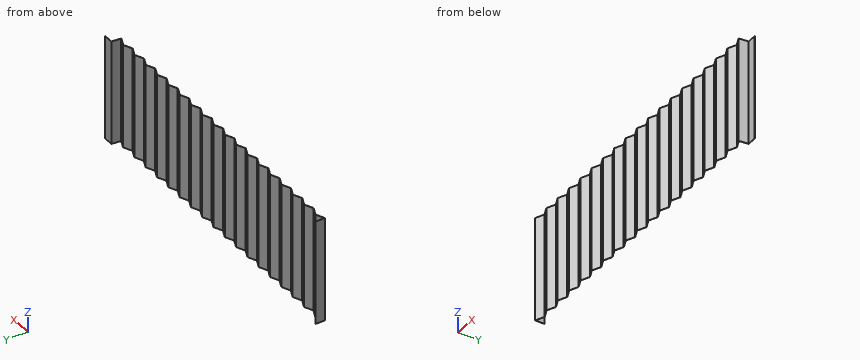
from build123d import *

# Parameters (mm, degrees)
EXTRUDE_THIN1_DEPTH = 85


with BuildPart() as part:
    # Sketch1 → Extrude-Thin1 (new, symmetric)
    with BuildSketch(Plane.XY):
        Polygon((0, 15.1), (0, 0), (13.79208513, 6.147226022), (27.58417026, 0), (41.37625539, 6.147226022), (55.16834052, 0), (68.960425651, 6.147226022), (82.752510781, 0), (96.544595911, 6.147226022), (110.336681041, 0), (124.128766171, 6.147226022), (137.920851301, 0), (151.712936431, 6.147226022), (165.505021561, 0), (179.297106692, 6.147226022), (193.089191822, 0), (206.881276952, 6.147226022), (220.673362082, 0), (234.465447212, 6.147226022), (248.257532342, 0), (262.049617472, 6.147226022), (275.841702602, 0), (289.633787732, 6.147226022), (303.425872863, 0), (317.217957993, 6.147226022), (331.010043123, 0), (344.802128253, 6.147226022), (358.594213383, 0), (372.386298513, 6.147226022), (386.178383643, 0), (399.970468773, 6.147226022), (413.762553904, 0), (427.554639034, 6.147226022), (441.346724164, 0), (455.138809294, 6.147226022), (468.930894424, 0), (482.722979554, 6.147226022), (496.515064684, 0), (498.249999842, 15), (513.249999842, 15), (513.249999842, 15.3), (497.982698545, 15.3), (496.263996817, 0.440351902), (482.722979554, 6.475675271), (468.930894424, 0.328449249), (455.138809294, 6.475675271), (441.346724164, 0.328449249), (427.554639034, 6.475675271), (413.762553904, 0.328449249), (399.970468773, 6.475675271), (386.178383643, 0.328449249), (372.386298513, 6.475675271), (358.594213383, 0.328449249), (344.802128253, 6.475675271), (331.010043123, 0.328449249), (317.217957993, 6.475675271), (303.425872863, 0.328449249), (289.633787732, 6.475675271), (275.841702602, 0.328449249), (262.049617472, 6.475675271), (248.257532342, 0.328449249), (234.465447212, 6.475675271), (220.673362082, 0.328449249), (206.881276952, 6.475675271), (193.089191822, 0.328449249), (179.297106692, 6.475675271), (165.505021561, 0.328449249), (151.712936431, 6.475675271), (137.920851301, 0.328449249), (124.128766171, 6.475675271), (110.336681041, 0.328449249), (96.544595911, 6.475675271), (82.752510781, 0.328449249), (68.960425651, 6.475675271), (55.16834052, 0.328449249), (41.37625539, 6.475675271), (27.58417026, 0.328449249), (13.79208513, 6.475675271), (0.3, 0.462161286), (0.3, 15.1), align=None)
    extrude(amount=EXTRUDE_THIN1_DEPTH, both=True)


solid = part.part
Geometry check sheet. Reference: the model listing, model coordinates, mm. Give positions to 0.01 mm unless a question says otherwise; leave off trailing zeros. Order: outer loops, then holes, each group sorted by start corner. A loop starts at its lowest first (then second) coordinate and runs counter-clockwise, first axis right, second up.
1) Gauge pin test, flat ends, axial feed: pin 1 (12 mm diameter, centred on x = 270.5, z = 62, fed in from -Y); pin 2 (7.5 mm diameter, centred on y = 9.5, z = -22.5, fed in from +X); pin 3 (2 mm diameter, centred on x = 196, z = 46.5, fed in from +Y); pin 4 (5 mm diameter, centred on x = 456.5, z = 10.5, fed in from +Y). Record the tip position at first contact, or that the pin passes through.
Results are:
pin 1: stops at y = 0
pin 2: stops at x = 498.05
pin 3: stops at y = 2.07
pin 4: stops at y = 6.48
2) Cross-section at A-A (y = 11). Record the boundary of the cut face in (x, z), then the cut area to 3 significant figures.
Results are:
outline: (0, -85) - (0.3, -85) - (0.3, 85) - (0, 85) - close; (497.49, -85) - (497.79, -85) - (497.79, 85) - (497.49, 85) - close
area: 102 mm2
3) Cross-section at B-B (x = 143.5). Record the boundary of the cut face in (y, z), then the cut area to 3 significant figures.
Results are:
outline: (2.49, -85) - (2.82, -85) - (2.82, 85) - (2.49, 85) - close
area: 55.8 mm2
4) Material ranges on probe 1 along X at (y, z) = (6.75, -46); probe 2 along X at (y, z) = (13.25, 18.5); probe 3 along Y at (x, z) = (289.5, -47), recorded low to high.
Results are:
probe 1: x = 0 to 0.3, 496.99 to 497.3
probe 2: x = 0 to 0.3, 497.75 to 498.05
probe 3: y = 6.09 to 6.42
